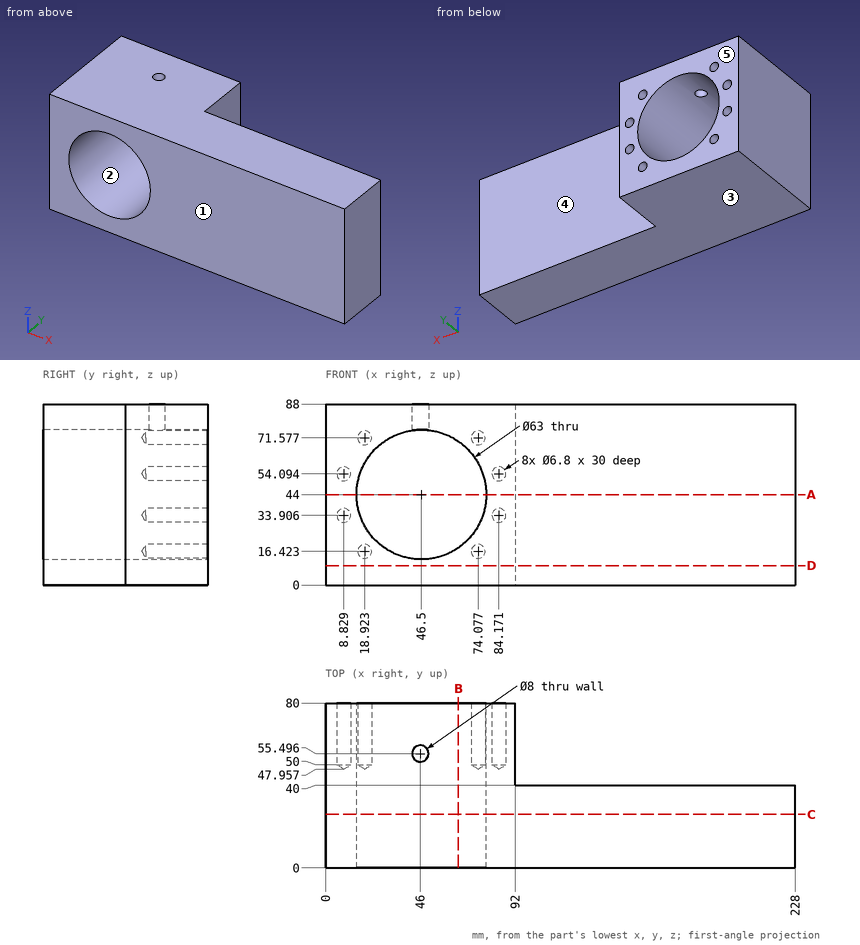
Job drawing, mm, ordinate dimensions from the low corner. One solid piece. A direction names the side the tool comes from. Give positions to 0.01 mm unless a question says otherwise; leave off trailing zeros. Write each loop counter-clockwise with the first axis right and the second up, starting at its lowest first coordinate (ties: lowest second). Pieces come first, ordered by that corner, then holes. Notation, with made-up numbers: M 6.5,-36.5 L 57.5,-36.5 A9 cw 57.5,-20.5 Z; hole C 50.5,31 d1. An arc over 180 degrees is marked long. One line per item, written item: value. Start each with the question number.
Q1. 3-axis set-ups, long thin cutter, end or side, ignore diameter. For the marked faces 4 and 5: which of +Z, -Z, +X, -X, +Y, -Y reach the whole face in a straight line?
Q2. Saw through at A-A, the plane z = 44. Write the cut outline in (x, y).
Q3. Saw through at B-B, the plane x = 64.5. Write the cut outline in (y, z).
Q4. Two-plate mould, pull along Z, no slides. Class the marked faces 1, 2 and 3: +Z half, -Z half, draft (parallel to the pull), parting line (faces both ways), or undercut.
Q5. Saw through at C-C, the plane y = 26. Write the cut outline in (x, z), plus the area to 3 significant figures.
Q6. Saw through at D-D, the plane z = 9.5. Write the cut outline in (x, y), plus the area to 3 significant figures.
Q7. Drop flat-ended pins along their axis: pin 1 Ø8 at (x, y) = (91, 32.5) entering from -Z; pin 2 Ø4 at (x, z) = (201, 63) entering from +Y; pin 3 Ø1.5 at (y, z) = (51.5, 60) entering from +X. Give the stop position or say it passes through.
Q8. Probe probe 1 along X at (y, z) = (56.5, 56) (1 decimal); probe 2 along X at (y, z) = (72, 11.5); probe 3 along Y at (x, z) = (170, 54.5). List the from-to ranges inside material, lowest first. Write a range as [from, to].
Output values:
1. face 4: +Z, -Z, +X, +Y
1. face 5: +Z, -Z, +X, -X, +Y
2. outline: M 0,0 L 15,0 L 15,80 L 0,80 Z; M 78,0 L 228,0 L 228,40 L 92,40 L 92,80 L 78,80 Z
3. outline: M 0,0 L 80,0 L 80,18.15 L 0,18.15 Z; M 0,69.85 L 80,69.85 L 80,88 L 0,88 Z
4. face 1: draft
4. face 2: undercut
4. face 3: -Z half
5. outline: M 0,0 L 228,0 L 228,88 L 0,88 Z; hole C 46.5,44 d63
5. area: 16,900 mm²
6. outline: M 0,0 L 228,0 L 228,40 L 92,40 L 92,80 L 0,80 Z
6. area: 12,800 mm²
7. pin 1: stops at z = 0
7. pin 2: stops at y = 40
7. pin 3: stops at x = 92
8. probe 1: x = [0, 6], [11.6, 17.4], [75.6, 81.4], [87, 92]
8. probe 2: x = [0, 92]
8. probe 3: y = [0, 40]
